Part model, mm, in its own coordinate system. Face numbers are marked on the shaded views. A direction names the side the tool comes from. Round coordinates to 2 decimals unless told otherwise and drop trailing zeros. Write each loop counter-clockwise with the first axis right and the second up, starting at its lowest first coordinate (ties: lowest second). Pieces come first, ordered by that corner, then holes. Notation, with made-up numbers: (-30, 72) -> (1, 72) arc R16 cw to (1, 97) -> close; hole circle Ø9 at (-27, 10). An arc over 180 degrees is marked (long way). Use CSV: the item, a comma, the result in double quotes. Start each with the question number.
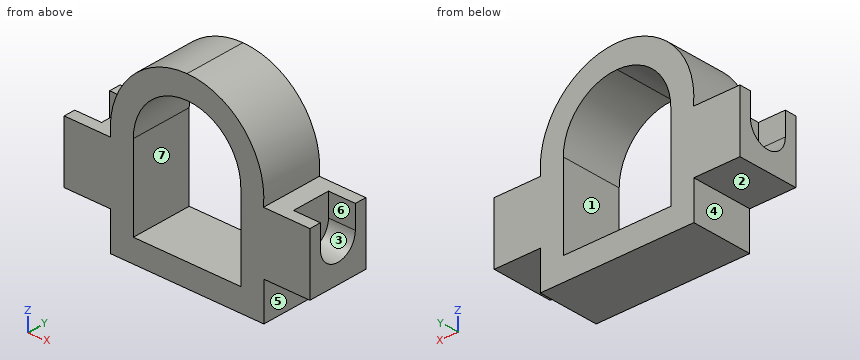
```python
from build123d import *

# Parameters (mm, degrees)
F1_DEPTH = 16
F3_DEPTH = 7


# Not quite as in the source:
# - a pattern or mirror of a feature is missing from the dataset's text; its kind, count and spacing are read off the source's solid


with BuildPart() as f1:
    # F0 (on Front) → F1 (new body)
    with BuildSketch(Plane.XZ):
        with BuildLine():
            Line((-20, 0), (0, 0))
            Line((0, 0), (0, 6))
            Line((0, 6), (-14, 6))
            Line((-14, 6), (-14, 28))
            ThreePointArc((-14, 28), (-9.8994949366, 37.8994949366), (0, 42))
            Line((0, 42), (0, 48))
            ThreePointArc((0, 48), (-14.8323969742, 41.416407865), (-19.8997487421, 26))
            Line((-19.8997487421, 26), (-32, 26))
            Line((-32, 26), (-32, 10))
            Line((-32, 10), (-20, 10))
            Line((-20, 10), (-20, 0))
        make_face()
    extrude(amount=F1_DEPTH)

    # F1_copies: F1 across plane


with BuildPart() as f1_1:
    add(f1.part)
    add(f1.part.mirror(Plane(origin=(0, 0, 0), x_dir=(0, 0, 1), z_dir=(1, 0, 0))))

    # F2 (on face) → F3 (cut)
    with BuildSketch(Plane(origin=(-32, 0, 0), x_dir=(0, -1, 0), z_dir=(-1, 0, 0))):
        with BuildLine():
            Line((13, 26), (3, 26))
            Line((3, 26), (3, 20))
            ThreePointArc((3, 20), (8, 15), (13, 20))
            Line((13, 20), (13, 26))
        make_face()
    f3 = extrude(amount=-F3_DEPTH, mode=Mode.SUBTRACT)

    # F3_copies: F3 across plane
    add(f3.mirror(Plane(origin=(0, 0, 0), x_dir=(0, 0, 1), z_dir=(1, 0, 0))), mode=Mode.SUBTRACT)


solid = f1_1.part
```
1. Flat gauge pins, fed straight in: pin 1 (8 mm diameter, centred on y = -10.5, z = 3.5, fed in from +X); pin 2 (5 mm diameter, centred on x = -21.5, y = -7, fed in from -Z); pin 3 (5 mm diameter, centred on x = 4.5, y = -7, fed in from +Z); pin 4 (9.5 mm diameter, centred on x = -28.5, y = -12, fed in from -Z). Where does each tip first touch, or does it go through?
2. Band-saw the part on B-B (y = -8). List the corners of the cut face in (x, z), then the cut area to 3 significant figures.
3. Pull direction Z, two halves, no side cores. Call the marked faces 1, 2 and 3: released by +Z, released by -Z, zero draft, split by the parting line, or undercut.
4. Band-saw the part on A-A (z = 8.5). List the corners of the cut face in (x, y), then the cut area to 3 significant figures.
5. Band-saw the part on C-C (x = 2.5). List the corners of the cut face in (y, z), then the cut area to 3 significant figures.
6. Band-saw the part on D-D (y = -11.75). List the corners of the cut face in (x, z), then the cut area to 3 significant figures.
7. Which spindle directions (+Z, -Z, +X, -X, +Y, -Y) get a long thin tool onto all of the face, cutting with end or side? Do the marked faces 4, 5, 6 and 7. Say none if no direction does.
8. Drill centre lines: line 1 along X through (y, z) = (-2.5, 18); line 2 along X through (y, z) = (-12.5, 25); line 3 along Z through (x, y) = (4, -10.5). Where is each one in solid material? Low to high. Write a range as [from, to].
Answers below:
1,pin 1,"stops at x = 20"
1,pin 2,"stops at z = 0"
1,pin 3,"stops at z = 47.9"
1,pin 4,"stops at z = 10"
2,outline,"(-32, 10) -> (-20, 10) -> (-20, 0) -> (20, 0) -> (20, 10) -> (32, 10) -> (32, 15) -> (25, 15) -> (25, 26) -> (19.9, 26) arc R20 ccw (long way) to (-19.9, 26) -> (-25, 26) -> (-25, 15) -> (-32, 15) -> close; hole (-14, 6) -> (14, 6) -> (14, 28) arc R14 ccw to (-14, 28) -> close"
2,area,"1,050 mm^2"
3,face 1,"undercut"
3,face 2,"released by -Z"
3,face 3,"released by +Z"
4,outline,"(-20, -16) -> (-14, -16) -> (-14, 0) -> (-20, 0) -> close; (14, -16) -> (20, -16) -> (20, 0) -> (14, 0) -> close"
4,area,"192 mm^2"
5,outline,"(-16, 0) -> (0, 0) -> (0, 6) -> (-16, 6) -> close; (-16, 41.77) -> (0, 41.77) -> (0, 47.84) -> (-16, 47.84) -> close"
5,area,"193 mm^2"
6,outline,"(-32, 10) -> (-20, 10) -> (-20, 0) -> (20, 0) -> (20, 10) -> (32, 10) -> (32, 16.69) -> (25, 16.69) -> (25, 26) -> (19.9, 26) arc R20 ccw (long way) to (-19.9, 26) -> (-25, 26) -> (-25, 16.69) -> (-32, 16.69) -> close; hole (-14, 6) -> (14, 6) -> (14, 28) arc R14 ccw to (-14, 28) -> close"
6,area,"1,080 mm^2"
7,face 4,"-Z, -X, +Y, -Y"
7,face 5,"-Z, +X, +Y, -Y"
7,face 6,"+Z, +X"
7,face 7,"+Y, -Y"
8,line 1,"x = [-32, -14], [14, 32]"
8,line 2,"x = [-25, -14], [14, 25]"
8,line 3,"z = [0, 6], [41.42, 47.6]"
